Verification items for the finished model (mm, model axes). Face numbers are marked on the shaded views. A direction names the side the tool comes from. Coordinates: 2 decimals unless noted, no trailing zeros. Order: outer loops, then holes, each group sorted by start corner. A loop starts at its lowest first (then second) coordinate and runs counter-clockwise, first axis right, second up. Notation, with made-up numbers: M 51,-40 L 67,-40 A5 cw 67,-34 Z; hole C -15.75,-29.75 d3. An arc over 180 degrees is marked long. Return JSON: item names as keys, results as strings.
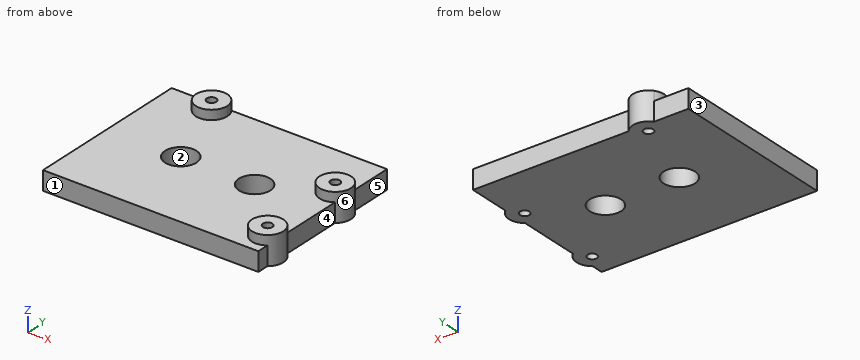
```python
from build123d import *
from build123d import SkipClean  # not in build123d's __all__

# Parameters (mm, degrees)
F0_R     = 5
F0_R_2   = 1.5
F1_DEPTH = 6
F2_R     = 1.5
F3_DEPTH = 3


# Not quite as in the source:
# - a feature names something its author has since deleted; it is built from what else it names


with BuildPart() as f1:
    # F0 (on Top) → F1 (new body)
    with BuildSketch(Plane.XY):
        with BuildLine():
            Line((42.65, 26.625), (11.4, 26.625))
            Line((11.4, 26.625), (-3.85, 26.625))
            ThreePointArc((-3.85, 26.625), (-7.85, 28.625), (-11.85, 26.625))
            Line((-11.85, 26.625), (-22.85, 26.625))
            Line((-22.85, 26.625), (-22.85, -26.625))
            Line((-22.85, -26.625), (45.65, -26.625))
            Line((45.65, -26.625), (45.65, -22.875))
            ThreePointArc((45.65, -22.875), (47.65, -18.875), (45.65, -14.875))
            Line((45.65, -14.875), (45.65, 5.125))
            ThreePointArc((45.65, 5.125), (47.65, 9.125), (45.65, 13.125))
            Line((45.65, 13.125), (45.65, 26.625))
            Line((45.65, 26.625), (42.65, 26.625))
        make_face()
        with Locations((0.5, 0)):
            Circle(F0_R, mode=Mode.SUBTRACT)
        with Locations((42.65, -18.875)):
            Circle(F0_R_2, mode=Mode.SUBTRACT)
        with BuildLine():
            ThreePointArc((29, 0), (24, -5), (19, 0))
            ThreePointArc((19, 0), (24, 5), (29, 0))
        make_face(mode=Mode.SUBTRACT)
        with BuildLine():
            ThreePointArc((-7.85, 25.125), (-6.7893398282, 24.6856601718), (-6.35, 23.625))
            ThreePointArc((-6.35, 23.625), (-8.9106601718, 22.5643398282), (-7.85, 25.125))
        make_face(mode=Mode.SUBTRACT)
        with Locations((42.65, 9.125)):
            Circle(F0_R_2, mode=Mode.SUBTRACT)
    extrude(amount=F1_DEPTH)

    # F2 (on face) → F3 (join)
    with BuildSketch(Plane.XY.offset(6)):
        with BuildLine():
            ThreePointArc((-11.85, 26.625), (-9.4311388301, 18.8815835097), (-2.85, 23.625))
            ThreePointArc((-2.85, 23.625), (-3.1065835097, 25.2061388301), (-3.85, 26.625))
            ThreePointArc((-3.85, 26.625), (-7.85, 28.625), (-11.85, 26.625))
        make_face()
        with Locations((-7.85, 23.625)):
            Circle(F2_R, mode=Mode.SUBTRACT)
        with BuildLine():
            ThreePointArc((47.65, 9.125), (47.122135955, 11.3610679775), (45.65, 13.125))
            ThreePointArc((45.65, 13.125), (37.65, 9.125), (45.65, 5.125))
            ThreePointArc((45.65, 5.125), (47.122135955, 6.8889320225), (47.65, 9.125))
        make_face()
        with Locations((42.65, 9.125)):
            Circle(F2_R, mode=Mode.SUBTRACT)
        with BuildLine():
            ThreePointArc((47.65, -18.875), (47.122135955, -16.6389320225), (45.65, -14.875))
            ThreePointArc((45.65, -14.875), (37.65, -18.875), (45.65, -22.875))
            ThreePointArc((45.65, -22.875), (47.122135955, -21.1110679775), (47.65, -18.875))
        make_face()
        with Locations((42.65, -18.875)):
            Circle(F2_R, mode=Mode.SUBTRACT)
    with SkipClean():  # cleaning this boolean's faces spoils the solid; the shape is the same uncleaned
        extrude(amount=F3_DEPTH)


solid = f1.part
```
Q1. Cross-section at D-D, the plane x = 42.65. Record the boundary of the cut face in (y, z) (3 decimals), and give its area (4 significant figures).
Values:
{"outline": "M -26.625,0 L -20.375,0 L -20.375,9 L -23.875,9 L -23.875,6 L -26.625,6 Z; M -17.375,0 L 7.625,0 L 7.625,9 L 4.125,9 L 4.125,6 L -13.875,6 L -13.875,9 L -17.375,9 Z; M 10.625,0 L 26.625,0 L 26.625,6 L 14.125,6 L 14.125,9 L 10.625,9 Z", "area": "325.5 mm^2"}
Q2. Cross-section at A-A, the plane x = 24. Record the boundary of the cut face in (y, z) (3 decimals).
Values:
{"outline": "M -26.625,0 L -5,0 L -5,6 L -26.625,6 Z; M 5,0 L 26.625,0 L 26.625,6 L 5,6 Z"}
Q3. Tool access check on the marked faces 4, 5 and 6. Record the directions out of +Z, -Z, +X, -X, +Y, -Y that give a thin tool (end or side, any length) a straight path to the whole face; none if there is none.
Values:
{"face 4": "+Z, -Z, +X", "face 5": "+Z, -Z, +X, +Y", "face 6": "+Z"}
Q4. Go/stop test with flat-tipped pins: pin 1 (3 mm diameter, centred on x = -0.5, y = 7, fed in from -Z); pin 2 (16 mm diameter, centred on x = 6, y = 0, fed in from +Z); pin 3 (4 mm diameter, centred on y = -25.5, z = 1.5, fed in from +X); pin 4 (3 mm diameter, centred on x = -20, z = 4, fed in from +Y) (3 decimals). Record where each tip stops, or that it passes through.
Values:
{"pin 1": "z = 0", "pin 2": "z = 6", "pin 3": "x = 45.65", "pin 4": "y = 26.625"}
Q5. Material ranges on line 1 along Y through (x, z) = (42.65, 6.5) (3 decimals); line 2 along Y through (x, z) = (42.65, 4.25) (3 decimals); line 3 along Y through (x, z) = (24, 4.65) (3 decimals), recorded low to high.
Values:
{"line 1": "-23.875 to -20.375, -17.375 to -13.875, 4.125 to 7.625, 10.625 to 14.125", "line 2": "-26.625 to -20.375, -17.375 to 7.625, 10.625 to 26.625", "line 3": "-26.625 to -5, 5 to 26.625"}
Q6. Cross-section at B-B, the plane z = 8.25. Record the boundary of the cut face in (x, y) (3 decimals), and give its area (3 significant figures).
Values:
{"outline": "C -7.85,23.625 d10; C 42.65,-18.875 d10; C 42.65,9.125 d10; hole C -7.85,23.625 d3; hole C 42.65,-18.875 d3; hole C 42.65,9.125 d3", "area": "214 mm^2"}
Q7. Draft check along Y on the marked faces 1, 2 and 3. Enter one of: pulls with the +Y half, pulls with the -Y half, needs draft (parallel to the pull), parting line crosses it, or undercut.
Values:
{"face 1": "pulls with the -Y half", "face 2": "undercut", "face 3": "needs draft"}
Q8. Cross-section at C-C, the plane y = 0. Record the boundary of the cut face in (x, z).
Values:
{"outline": "M -22.85,0 L -4.5,0 L -4.5,6 L -22.85,6 Z; M 5.5,0 L 19,0 L 19,6 L 5.5,6 Z; M 29,0 L 45.65,0 L 45.65,6 L 29,6 Z"}
